Here's the drawing with two shaded views (mm, measured from the low corner). I have some questions. Coordinates: 2 decimals unless noted, no trailing zeros. Order: outer loops, then holes, each group sorted by start corner. A loop starts at its lowest first (then second) coordinate and runs counter-clockwise, first axis right, second up. Notation, with made-up numbers: (59, 70) -> (76, 70) arc R3 ccw to (76, 74) -> close; hole circle Ø2 at (2, 71.5). An arc over 180 degrees is marked (long way). Answer as a JSON object with one key per item and string values. Group by question number.
(1) I need wall thicknesses on line 1 (X direction, y = 2, z = 8.5) (1 decimal); line 2 (Y direction, x = 3.5, z = 8.25) (1 decimal); line 3 (Z direction, x = 3.75, y = 2.5). Which ranges of each line are inside material? Lowest first, please.
(2) If we mould it in two halves opening along X, with no side actions, what happens to the marked faces 1, 2, 3 and 4? For each: pulls with the +X half, pulls with the -X half, needs draft (parallel to the pull), parting line crosses it, or undercut.
(3) I want a section at B-B, the plane x = 3.5. List the corners of the cut face in (y, z) for me (1 decimal).
(4) I want a section at A-A, the plane y = 3.25. List the corners of the cut face in (x, z) for me (1 decimal), plus the area to 3 significant figures.
(5) I want a section at C-C, the plane z = 36. List the corners of the cut face in (x, y) for me (1 decimal).
(6) I want a section at D-D, the plane x = 22.5. List the corners of the cut face in (y, z) for me (1 decimal).
(7) For pin 1 (3 mm diameter, centred on x = 22.5, y = 3.005, fed in from +Z), with a flat end and sliding along its axis, tell me the tip position at first contact or that it passes through.
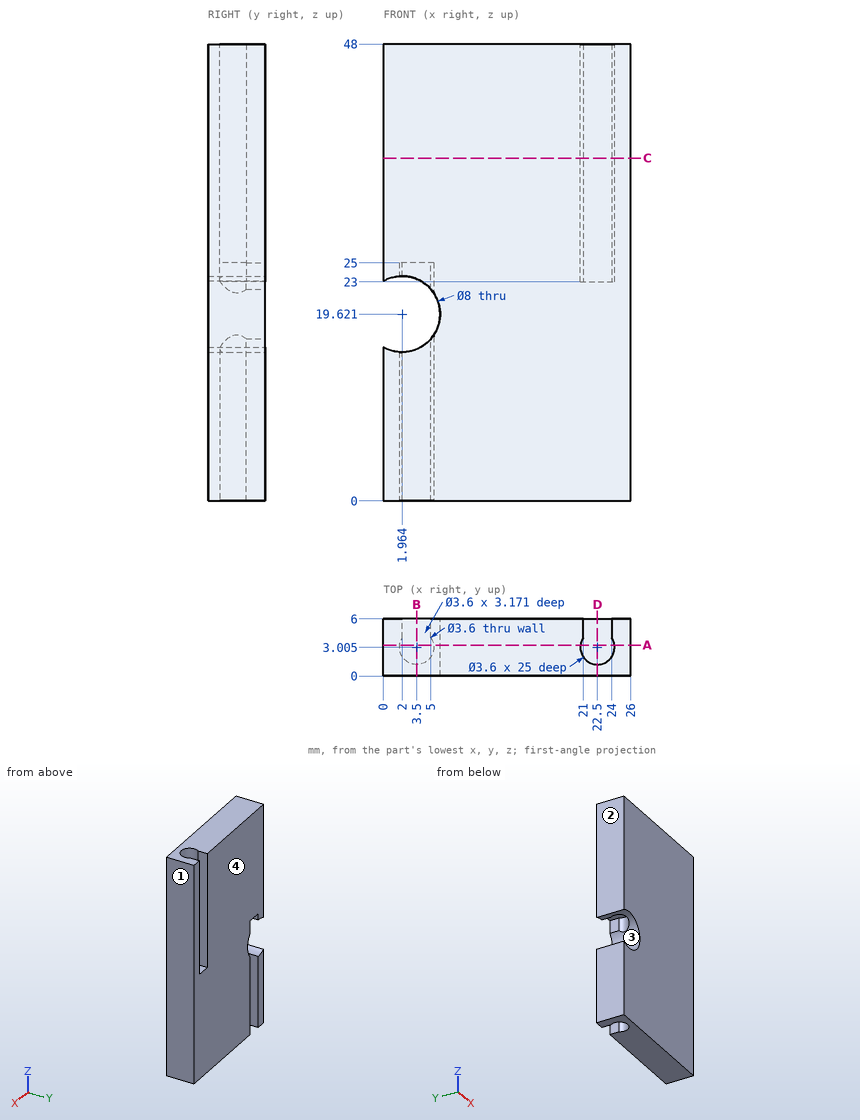
Computed values:
{
 "1": {"line 1": "x = 0 to 2, 5 to 26", "line 2": "y = 0 to 1.2", "line 3": "z = 25 to 48"},
 "2": {"face 1": "pulls with the +X half", "face 2": "pulls with the -X half", "face 3": "undercut", "face 4": "needs draft"},
 "3": {"outline": "(0, 0) -> (1.2, 0) -> (1.2, 15.9) -> (0, 15.9) -> close; (0, 23.3) -> (1.2, 23.3) -> (1.2, 25) -> (6, 25) -> (6, 48) -> (0, 48) -> close"},
 "4": {"outline": "(0, 0) -> (1.7, 0) -> (1.7, 15.6) arc R4 cw to (0, 16.1) -> close; (0, 23.1) arc R4 cw to (1.7, 23.6) -> (1.7, 25) -> (5.3, 25) -> (5.3, 21.9) arc R4 cw to (5.3, 17.4) -> (5.3, 0) -> (26, 0) -> (26, 48) -> (24.3, 48) -> (24.3, 23) -> (20.7, 23) -> (20.7, 48) -> (0, 48) -> close", "area": "1,050 mm2"},
 "5": {"outline": "(0, 0) -> (26, 0) -> (26, 6) -> (24, 6) -> (24, 4) arc R1.8 cw (long way) to (21, 4) -> (21, 6) -> (0, 6) -> close"},
 "6": {"outline": "(0, 0) -> (6, 0) -> (6, 23) -> (1.2, 23) -> (1.2, 48) -> (0, 48) -> close"},
 "7": {"pin 1": "stops at z = 23"}
}
